Can you work these out from the drawing? Everything is in mm from the part's minimum corner. Coordinates: 2 decimals unless noted, no trailing zeros. Write each loop counter-clockwise with the first axis right and the second up, starting at its lowest first coordinate (ties: lowest second). Pieces come first, ordered by that corner, then holes.
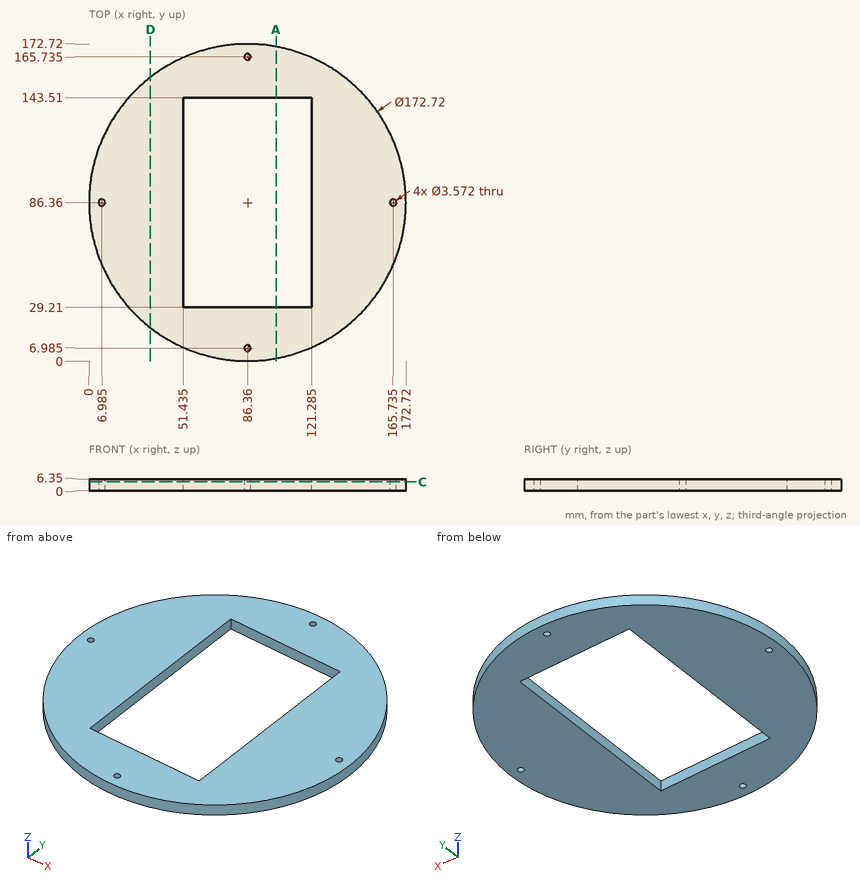
1. I want a section at D-D (x = 33.5). List the corners of the cut face in (y, z) for me.
2. I want a section at A-A (x = 102). List the corners of the cut face in (y, z) for me.
3. I want a section at C-C (z = 4.75). List the corners of the cut face in (x, y) for me (3 decimals).
4. For pin 1 Ø2 at (x, z) = (76.5, 2.5) entering from +Y; pin 2 Ø4 at (x, y) = (86.36, 6.985) entering from -Z; pin 3 Ø3 at (y, z) = (139.5, 5) entering from -X; pin 4 Ø1.5 at (x, z) = (137, 2.5) entering from +Y, each with a flat end and sliding along its axis, tell me the tip position at first contact or that it passes through.
5. If I drill on line 1 (Y direction, x = 86.36, z = 2); line 2 (X direction, y = 94, z = 6) (1 decimal); line 3 (X direction, y = 30.5, z = 3) (1 decimal), over which ranges is the centre line in solid material (lowest first)?
Response values:
1. outline: (18.07, 0) - (154.65, 0) - (154.65, 6.35) - (18.07, 6.35) - close
2. outline: (1.43, 0) - (29.21, 0) - (29.21, 6.35) - (1.43, 6.35) - close; (143.51, 0) - (171.29, 0) - (171.29, 6.35) - (143.51, 6.35) - close
3. outline: circle Ø172.72 at (86.36, 86.36); hole circle Ø3.572 at (6.985, 86.36); hole (51.435, 29.21) - (121.285, 29.21) - (121.285, 143.51) - (51.435, 143.51) - close; hole circle Ø3.572 at (86.36, 6.985); hole circle Ø3.572 at (86.36, 165.735); hole circle Ø3.572 at (165.735, 86.36)
4. pin 1: stops at y = 172.26
4. pin 2: stops at z = 0
4. pin 3: stops at x = 17.14
4. pin 4: stops at y = 156.85
5. line 1: y = 0 to 5.2, 8.77 to 29.21, 143.51 to 163.95, 167.52 to 172.72
5. line 2: x = 0.3 to 51.4, 121.3 to 172.4
5. line 3: x = 20.5 to 51.4, 121.3 to 152.2
